```python
from build123d import *

# Parameters (mm, degrees)
SKETCH1_R           = 17.5
SKETCH1_R_2         = 1.5
BOSS_EXTRUDE1_DEPTH = 10
SKETCH2_R           = 9
BOSS_EXTRUDE2_DEPTH = 30
SKETCH2_2_R         = 9
CUT_EXTRUDE1_DEPTH  = 39.890872965
FILLET1_R           = 4
SKETCH4_4_W         = 1.75
SKETCH4_4_H         = 11.757944022


with BuildPart() as part:
    # Sketch1 → Boss-Extrude1 (new body)
    with BuildSketch(Plane.XY):
        Circle(SKETCH1_R)
        with Locations((0, 13.5)):
            Circle(SKETCH1_R_2, mode=Mode.SUBTRACT)
        with Locations((11.691342951, -6.75)):
            Circle(SKETCH1_R_2, mode=Mode.SUBTRACT)
        with Locations((-11.691342951, -6.75)):
            Circle(SKETCH1_R_2, mode=Mode.SUBTRACT)
    extrude(amount=BOSS_EXTRUDE1_DEPTH)

    # Sketch2 → Boss-Extrude2 (add)
    with BuildSketch(Plane.XY.offset(10)):
        with BuildLine():
            ThreePointArc((10.71198615, -4.18370084), (9.959292144, 5.75), (1.732801866, 11.368702551))
            ThreePointArc((1.732801866, 11.368702551), (0, 10.753177996), (-1.732801866, 11.368702551))
            ThreePointArc((-1.732801866, 11.368702551), (-9.959292144, 5.75), (-10.71198615, -4.18370084))
            ThreePointArc((-10.71198615, -4.18370084), (-9.312525316, -5.376588998), (-8.979184285, -7.185001711))
            ThreePointArc((-8.979184285, -7.185001711), (0, -11.5), (8.979184285, -7.185001711))
            ThreePointArc((8.979184285, -7.185001711), (9.312525316, -5.376588998), (10.71198615, -4.18370084))
        make_face()
        Circle(SKETCH2_R, mode=Mode.SUBTRACT)
    extrude(amount=BOSS_EXTRUDE2_DEPTH)

    # Sketch2<2> → Cut-Extrude1 (cut, through all)
    with BuildSketch(Plane.XY.offset(10)):
        Circle(SKETCH2_2_R)
    extrude(amount=-CUT_EXTRUDE1_DEPTH, mode=Mode.SUBTRACT)

    # Fillet1
    # the kernel refuses this fillet: 4 mm, written as the material it adds along each edge
    with BuildSketch(Plane(origin=(0, 0, 10), x_dir=(-0.9810153845306142, 0.19392992372053186, 0), z_dir=(0.19392992372053186, 0.9810153845306142, 0))) as fillet1_piece_1_section:
        with BuildLine():
            CenterArc((11.5 + FILLET1_R, FILLET1_R), FILLET1_R, 180, 90)
            Line((11.5, FILLET1_R), (11.5, 0))
            Line((11.5, 0), (11.5 + FILLET1_R, 0))
        make_face()
    fillet1_piece_1 = revolve(axis=Axis((0, 0, 10), (0, 0, 1)), revolution_arc=202.364438996, mode=Mode.PRIVATE)
    fillet1_piece_1 = fillet1_piece_1 - Plane(origin=(11.691342951, -6.75, 10.886663102), x_dir=(-0.9873805666072768, -0.15836545294442564, 0), z_dir=(0, 0, -1)) * Cylinder(2.746822004, 62, mode=Mode.PRIVATE)
    fillet1_piece_1 = fillet1_piece_1 - Plane(origin=(-11.691342951, -6.75, 10.886663102), x_dir=(0.3565417779714824, 0.9342793803573609, 0), z_dir=(0, 0, -1)) * Cylinder(2.746822004, 62, mode=Mode.PRIVATE)
    add(fillet1_piece_1)
    with BuildSketch(Plane(origin=(0, 0, 10), x_dir=(0.3225594517692616, -0.9465492063671669, 0), z_dir=(-0.9465492063671669, -0.3225594517692616, 0))) as fillet1_piece_2_section:
        with BuildLine():
            CenterArc((11.5 + FILLET1_R, FILLET1_R), FILLET1_R, 180, 90)
            Line((11.5, FILLET1_R), (11.5, 0))
            Line((11.5, 0), (11.5 + FILLET1_R, 0))
        make_face()
    fillet1_piece_2 = revolve(axis=Axis((0, 0, 10), (0, 0, 1)), revolution_arc=202.364438996, mode=Mode.PRIVATE)
    fillet1_piece_2 = fillet1_piece_2 - Plane(origin=(11.691342951, -6.75, 10.886663102), x_dir=(-0.9873805666072768, -0.15836545294442564, 0), z_dir=(0, 0, -1)) * Cylinder(2.746822004, 62, mode=Mode.PRIVATE)
    fillet1_piece_2 = fillet1_piece_2 - Plane(origin=(0, 13.5, 10.886663102), x_dir=(0.6308387886354789, -0.7759139274126491, 0), z_dir=(0, 0, -1)) * Cylinder(2.746822004, 62, mode=Mode.PRIVATE)
    add(fillet1_piece_2)
    with BuildSketch(Plane(origin=(0, 0, 10), x_dir=(0.6584559327613483, 0.7526192826465335, 0), z_dir=(0.7526192826465335, -0.6584559327613483, 0))) as fillet1_piece_3_section:
        with BuildLine():
            CenterArc((11.5 + FILLET1_R, FILLET1_R), FILLET1_R, 180, 90)
            Line((11.5, FILLET1_R), (11.5, 0))
            Line((11.5, 0), (11.5 + FILLET1_R, 0))
        make_face()
    fillet1_piece_3 = revolve(axis=Axis((0, 0, 10), (0, 0, 1)), revolution_arc=202.364438996, mode=Mode.PRIVATE)
    fillet1_piece_3 = fillet1_piece_3 - Plane(origin=(0, 13.5, 10.886663102), x_dir=(0.6308387886354789, -0.7759139274126491, 0), z_dir=(0, 0, -1)) * Cylinder(2.746822004, 63, mode=Mode.PRIVATE)
    fillet1_piece_3 = fillet1_piece_3 - Plane(origin=(-11.691342951, -6.75, 10.886663102), x_dir=(0.3565417779714824, 0.9342793803573609, 0), z_dir=(0, 0, -1)) * Cylinder(2.746822004, 63, mode=Mode.PRIVATE)
    add(fillet1_piece_3)

    # Sketch4 → Cut-Revolve1 (revolve, cut)
    with BuildSketch(Plane.XY.offset(30), mode=Mode.PRIVATE) as cut_revolve1_sk:
        Polygon((-16.858526531, 9.733274831), (-6.675848312, 3.85430282), (-7.550848312, 2.338758363), (-17.733526531, 8.217730374), align=None)
    revolve(cut_revolve1_sk.sketch.rotate(Axis((0, 0, 30), (-0.8660254037844364, 0.5000000000000039, 0)), 180), axis=Axis((0, 0, 30), (-0.8660254037844364, 0.5000000000000039, 0)), mode=Mode.SUBTRACT)

    # Sketch4<3> → Cut-Revolve2 (revolve, cut)
    with BuildSketch(Plane.XY.offset(30), mode=Mode.PRIVATE) as cut_revolve2_sk:
        Polygon((15.983526531, 11.248819288), (16.858526531, 9.733274831), (6.675848312, 3.85430282), (5.800848312, 5.369847276), align=None)
    revolve(cut_revolve2_sk.sketch.rotate(Axis((0, 0, 30), (0.8660254037844362, 0.5000000000000044, 0)), 180), axis=Axis((0, 0, 30), (0.8660254037844362, 0.5000000000000044, 0)), mode=Mode.SUBTRACT)

    # Sketch4<4> → Cut-Revolve3 (revolve, cut)
    with BuildSketch(Plane.XY.offset(30), mode=Mode.PRIVATE) as cut_revolve3_sk:
        with Locations((0.875, -13.587577651)):
            Rectangle(SKETCH4_4_W, SKETCH4_4_H)
    revolve(cut_revolve3_sk.sketch.rotate(Axis((0, 0, 30), (0, -1, 0)), 90), axis=Axis((0, 0, 30), (0, -1, 0)), mode=Mode.SUBTRACT)


solid = part.part
```
CAD build for the part. Positions are in the model's coordinates, mm. A direction names the side the tool comes from. Coordinates: 2 decimals unless noted, no trailing zeros. Write each loop counter-clockwise with the first axis right and the second up, starting at its lowest first coordinate (ties: lowest second). Pieces come first, ordered by that corner, then holes.
(1) Two-plate mould, pull along Z, no slides. Class faces 1 (the face through (-0.08, -10.15, 28.25)), 2 (the face through (8, -8, 0)), 3 (the face through (-13.887, -10.648, 4.93)), 4 (the face through (-8.01, 6.49, 30.67)): +Z half, -Z half, draft (parallel to the pull), parting line (faces both ways), or undercut.
(2) Flat gauge pins, fed straight in: pin 1 (4 mm diameter, centred on x = 0, y = 13.5, fed in from -Z); pin 2 (1 mm diameter, centred on x = -5, y = -13.5, fed in from +Z); pin 3 (8 mm diameter, centred on y = 12.5, z = 23, fed in from +X); pin 4 (5 mm diameter, centred on x = 11.69, y = -6.75, fed in from +Z). Where does each tip first touch, or does it go through?
(3) 3-axis set-ups, long thin cutter, end or side, ignore diameter. For faces 5 (the face through (-0.1, -11.5, 26.8)), 6 (the face through (10.031, 5.625, 26.818)), 7 (the face through (-10, -5, 10)), 8 (the face through (-9.89, 5.87, 26.82)): which of +Z, -Z, +X, -X, +Y, -Y reach the whole face in a straight line?
(4) Cut at A-A, the plane y = 0. List the corners of the cut face in (x, z), and give its area (3 significant figures).
(5) Drill centre lines: probe 1 along Y at (x, z) = (0, 6); probe 2 along X at (y, z) = (-0.5, 8); probe 3 along X at (y, z) = (-3.5, 37). Where is each one in solid material? Low to high.
(6) Cut at C-C, the plane z = 34. List the corners of the cut face in (x, y) (3 decimals), and give its area (3 significant figures).
(7) Cut at B-B, the plane z = 2. List the corners of the cut face in (x, y).
Geometry says:
1. face 1: undercut
1. face 2: -Z half
1. face 3: draft
1. face 4: undercut
2. pin 1: stops at z = 0
2. pin 2: stops at z = 10.34
2. pin 3: stops at x = 7.75
2. pin 4: stops at z = 10
3. face 5: +Z, -Y
3. face 6: +Z, +X
3. face 7: +Z
3. face 8: +Z, -X
4. outline: (-17.5, 0) - (-9, 0) - (-9, 40) - (-11.5, 40) - (-11.5, 14) arc R4 cw to (-15.5, 10) - (-17.5, 10) - close; (9, 0) - (17.5, 0) - (17.5, 10) - (15.5, 10) arc R4 cw to (11.5, 14) - (11.5, 40) - (9, 40) - close
4. area: 327 mm2
5. probe 1: y = -17.5 to -9, 9 to 12, 15 to 17.5
5. probe 2: x = -17.49 to -8.99, 8.99 to 17.49
5. probe 3: x = -10.95 to -8.29, 8.29 to 10.95
6. outline: (-10.712, -4.184) arc R2.747 cw to (-8.979, -7.185) arc R11.5 ccw to (8.979, -7.185) arc R2.747 cw to (10.712, -4.184) arc R11.5 ccw to (1.733, 11.369) arc R2.747 cw to (-1.733, 11.369) arc R11.5 ccw to start; hole circle Ø18 at (0, 0)
6. area: 156 mm2
7. outline: circle Ø35 at (0, 0); hole circle Ø3 at (-11.69, -6.75); hole circle Ø18 at (0, 0); hole circle Ø3 at (0, 13.5); hole circle Ø3 at (11.69, -6.75)
